Read the model definition and answer for the solid it produces. Units are mm, in the model's axes. A direction names the side the tool comes from. Coordinates: 2 decimals unless noted, no trailing zeros. Write each loop counter-clockwise with the first axis right and the second up, starting at its lowest first coordinate (ties: lowest second). Pieces come first, ordered by that corner, then holes. Notation, with made-up numbers: (66.25, -18.75) -> (122.25, -18.75) arc R32 ccw to (122.25, 13.25) -> close; hole circle Ø2 at (-27.5, -33.5). An arc over 180 degrees is marked (long way). Write item = value, one per line. Start each with the question number.
1) Section A-A (x = -24.7) is taken. Determine the outline of the cut face in (y, z).
2) Section C-C (x = -10) is taken. Determine the outline of the cut face in (y, z).
3) Find the intervals of material crossed by line 1 along Z through (x, y) = (24.8, 28.6); line 2 along Z through (x, y) = (24, 28); line 3 along X through (y, z) = (10.5, -9), in increasing order. Write a range as from..to.
4) A tool of negligible diameter and unlimited length cuts with its end or side. For faces 5 (the face through (-22, 11, 0)), 6 (the face through (-20.05, 34, 0)), 7 (the face through (-22, 9, 4)), 8 (the face through (24, 27.3, 0)), 9 (the face through (-22, 7, 0)), from which of +Z, -Z, +X, -X, +Y, -Y can it reach the whole face along a straight path? Write none if from no direction.
5) For a pull along Z with two mould halves and no side action, classify faces 1 (the face through (20.05, 34, 0)), 2 (the face through (22.55, 28.67, -5.09)), 3 (the face through (-12.4, 41.5, 1.8)), 4 (the face through (-22, 9, -4)) as released by +Z, released by -Z, zero draft, split by the parting line, or undercut.
6) Section D-D (y = 23.5) is taken. Determine the outline of the cut face in (x, z).
7) Flat-ended cylindrical pins translate along their axes: pin 1 Ø3 at (x, z) = (12, 8) entering from -Y; pin 2 Ø1.5 at (x, z) = (12, 2.5) entering from +Y; pin 3 Ø3.5 at (x, z) = (-25, 4) entering from -Y; pin 4 Ø10 at (y, z) = (13, -3) entering from +X. Find the tip coordinate at first contact, or state that the pin passes through.
8) Section B-B (y = 10) is taken. Determine the outline of the cut face in (x, z), plus the area to 3 significant figures.
from build123d import *

# Parameters (mm, degrees)
SKETCH_1_W          = 40.1
SKETCH_1_H          = 20.1
EXTRUDE_2_DEPTH     = 38.8
SKETCH_2_W          = 54
SKETCH_2_H          = 20.1
EXTRUDE_3_DEPTH     = 2.7
SKETCH_4_R          = 3
EXTRUDE_4_DEPTH     = 5.45
SKETCH_5_R          = 2.25
CUT_EXTRUDE_1_DEPTH = 31
SKETCH_6_W          = 8
SKETCH_6_H          = 4
EXTRUDE_5_DEPTH     = 3


with BuildPart() as part:
    # ｽｹｯﾁ1 → ﾎﾞｽ - 押し出し2 (new body)
    with BuildSketch(Plane(origin=(0, 0, 0), x_dir=(1, 0, 0), z_dir=(0, 1, 0))):
        Rectangle(SKETCH_1_W, SKETCH_1_H)
    extrude(amount=EXTRUDE_2_DEPTH)

    # ｽｹｯﾁ2 → ﾎﾞｽ - 押し出し3 (add)
    with BuildSketch(Plane(origin=(0, 30, 0), x_dir=(-1, 0, 0), z_dir=(0, -1, 0))):
        Rectangle(SKETCH_2_W, SKETCH_2_H)
    extrude(amount=EXTRUDE_3_DEPTH)

    # ｽｹｯﾁ4 → ﾎﾞｽ - 押し出し4 (add)
    with BuildSketch(Plane(origin=(0, 38.8, 0), x_dir=(1, 0, 0), z_dir=(0, 1, 0))):
        with Locations((-10, 0)):
            Circle(SKETCH_4_R)
    extrude(amount=EXTRUDE_4_DEPTH)

    # ｽｹｯﾁ5 → ｶｯﾄ - 押し出し1 (cut, through all)
    with BuildSketch(Plane(origin=(0, 30, 0), x_dir=(1, 0, 0), z_dir=(0, 1, 0))):
        with Locations((24.8, 5)):
            Circle(SKETCH_5_R)
        with Locations((24.8, -5)):
            Circle(SKETCH_5_R)
        with Locations((-24.7, 5)):
            Circle(SKETCH_5_R)
        with Locations((-24.7, -5)):
            Circle(SKETCH_5_R)
    extrude(amount=-CUT_EXTRUDE_1_DEPTH, mode=Mode.SUBTRACT)

    # ｽｹｯﾁ6 → ﾎﾞｽ - 押し出し5 (add)
    with BuildSketch(Plane.ZY.offset(20.05)):
        with Locations((0, 9)):
            Rectangle(SKETCH_6_W, SKETCH_6_H)
    extrude(amount=EXTRUDE_5_DEPTH)


solid = part.part
Answer key:
q1.outline = (27.3, -10.05) -> (30, -10.05) -> (30, -7.25) -> (27.3, -7.25) -> close; (27.3, -2.75) -> (30, -2.75) -> (30, 2.75) -> (27.3, 2.75) -> close; (27.3, 7.25) -> (30, 7.25) -> (30, 10.05) -> (27.3, 10.05) -> close
q2.outline = (0, -10.05) -> (38.8, -10.05) -> (38.8, -3) -> (44.25, -3) -> (44.25, 3) -> (38.8, 3) -> (38.8, 10.05) -> (0, 10.05) -> close
q3.line_1 = -10.05..-7.25, -2.75..2.75, 7.25..10.05
q3.line_2 = -10.05..-7.1, -2.9..2.9, 7.1..10.05
q3.line_3 = -20.05..20.05
q4.face_5 = +Z, -Z, -X
q4.face_6 = +Z, -Z, -X, +Y
q4.face_7 = +Z, -X, -Y
q4.face_8 = +Z, -Z, +X, -Y
q4.face_9 = +Z, -Z, -X, -Y
q5.face_1 = zero draft
q5.face_2 = undercut
q5.face_3 = split by the parting line
q5.face_4 = released by -Z
q6.outline = (-20.05, -10.05) -> (20.05, -10.05) -> (20.05, 10.05) -> (-20.05, 10.05) -> close
q7.pin_1 = 0
q7.pin_2 = 38.8
q7.pin_3 = 27.3
q7.pin_4 = 20.05
q8.outline = (-23.05, -4) -> (-20.05, -4) -> (-20.05, -10.05) -> (20.05, -10.05) -> (20.05, 10.05) -> (-20.05, 10.05) -> (-20.05, 4) -> (-23.05, 4) -> close
q8.area = 830 mm^2
